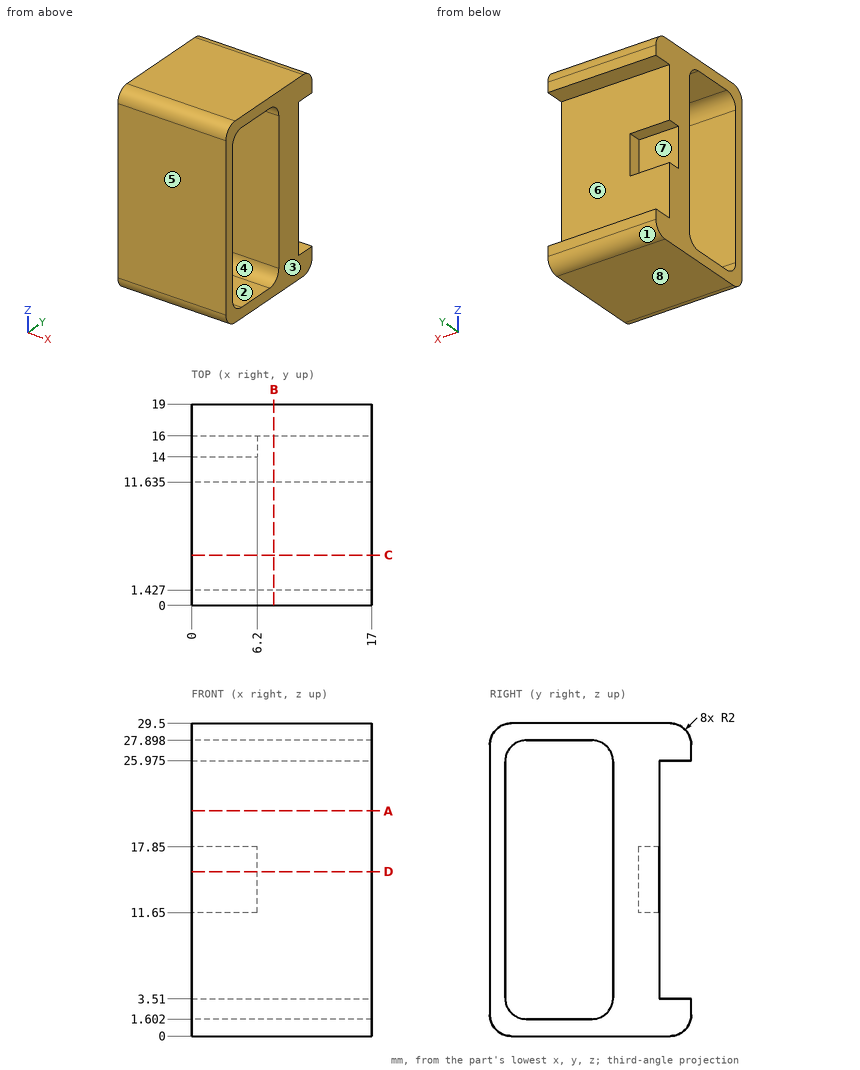
Source: three-view drawing plus pictorial views. Frame: mm from the lowest corner of the part. A direction names the side the tool comes from. Give positions to 0.01 mm unless a question says otherwise; leave off trailing zeros. Order: outer loops, then holes, each group sorted by start corner. A loop starts at its lowest first (then second) coordinate and runs counter-clockwise, first axis right, second up. Notation, with made-up numbers: (40, 55.5) -> (78, 55.5) arc R24 ccw to (78, 68.5) -> close; hole circle Ø10 at (8, -35). An arc over 180 degrees is marked (long way). Put each result on its own line as item: value.
Q1. Section D-D, the plane z = 15.5. Return loops of the section in (x, y) (1 decimal).
Here are the results:
outline: (0, 0) -> (17, 0) -> (17, 1.4) -> (0, 1.4) -> close; (0, 11.6) -> (17, 11.6) -> (17, 16) -> (6.2, 16) -> (6.2, 14) -> (0, 14) -> close
Q2. Section A-A, the plane z = 21.25. Return loops of the section in (x, y) (1 decimal).
Here are the results:
outline: (0, 0) -> (17, 0) -> (17, 1.4) -> (0, 1.4) -> close; (0, 11.6) -> (17, 11.6) -> (17, 16) -> (0, 16) -> close
Q3. Section B-B, the plane x = 7.75. Return loops of the section in (y, z) (1 decimal).
Here are the results:
outline: (0, 2) arc R2 ccw to (2, 0) -> (17, 0) arc R2 ccw to (19, 2) -> (19, 3.5) -> (16, 3.5) -> (16, 26) -> (19, 26) -> (19, 27.5) arc R2 ccw to (17, 29.5) -> (2, 29.5) arc R2 ccw to (0, 27.5) -> close; hole (1.4, 3.6) arc R2 ccw to (3.4, 1.6) -> (9.6, 1.6) arc R2 ccw to (11.6, 3.6) -> (11.6, 25.9) arc R2 ccw to (9.6, 27.9) -> (3.4, 27.9) arc R2 ccw to (1.4, 25.9) -> close
Q4. Draft query along Z for the marked faces 1, 2 and 3. Return one class per face: released by +Z, released by -Z, zero draft, split by the parting line, or undercut.
Here are the results:
face 1: released by -Z
face 2: undercut
face 3: zero draft
Q5. Section C-C, the plane y = 4.75. Return loops of the section in (x, z).
Here are the results:
outline: (0, 0) -> (17, 0) -> (17, 1.6) -> (0, 1.6) -> close; (0, 27.9) -> (17, 27.9) -> (17, 29.5) -> (0, 29.5) -> close
Q6. Reachability of the marked faces 4, 5, 6, 7 and 8 from +Z, -Z, +X, -X, +Y, -Y: full face, straight path, thin tool, end or side. Return the list, or none.
Here are the results:
face 4: +X, -X
face 5: +Z, -Z, +X, -X, -Y
face 6: +X, -X, +Y
face 7: -X, +Y
face 8: -Z, +X, -X, +Y, -Y
Q7. Pin query (flat end, axial travel): pin 1 (1.5 mm diameter, centred on x = 12, y = 18, fed in from -Z); pin 2 (5 mm diameter, centred on x = 14, z = 17.5, fed in from +Y); pin 3 (3 mm diameter, centred on x = 2.5, z = 14, fed in from +Y). Return the tip coordinate at first contact, or that it passes through.
Here are the results:
pin 1: stops at z = 0.02
pin 2: stops at y = 16
pin 3: stops at y = 14
Q8. Material intervals for L1, parallel to Y at x = 2.25, z = 18.25 (1 decimal); L2, parallel to Z at x = 6.75, y = 3.5; L3, parallel to Y at x = 5.75, z = 12.5 (1 decimal), sorted ascending.
Here are the results:
L1: y = 0 to 1.4, 11.6 to 16
L2: z = 0 to 1.6, 27.9 to 29.5
L3: y = 0 to 1.4, 11.6 to 14
